Drawing for the job (mm, zero at the part's lowest x, y, z). A direction names the side the tool comes from. Round coordinates to 2 decimals unless told otherwise and drop trailing zeros. Write each loop counter-clockwise with the first axis right and the second up, starting at its lowest first coordinate (ties: lowest second). Pieces come first, ordered by that corner, then holes. Notation, with made-up numbers: (-33.5, -21) -> (23.5, -21) arc R11 cw to (23.5, -8) -> close; hole circle Ø5 at (-35, 40). An arc over 180 degrees is marked (long way). One line per question, with ' | ' between items.
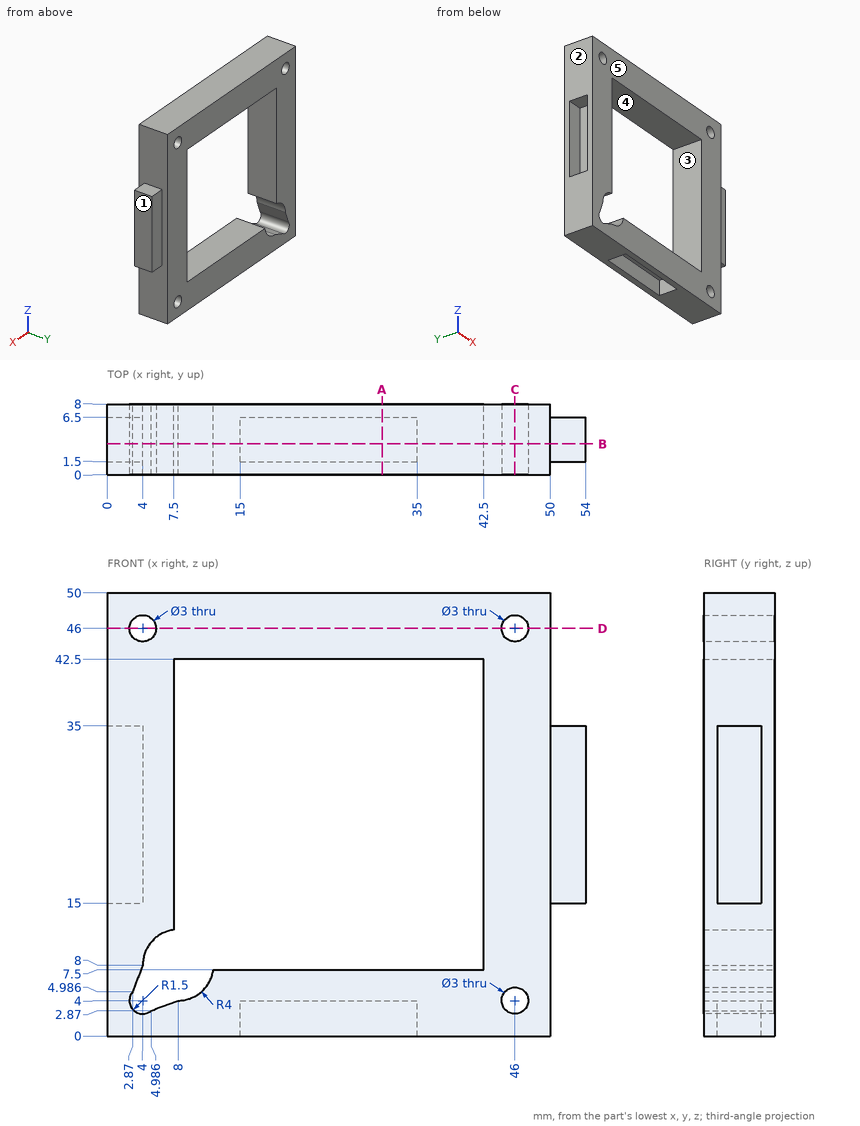
(1) Drop flat-ended pins along their axis: pin 1 (1.5 mm diameter, centred on y = 2, z = 13.5, fed in from +X); pin 2 (1.2 mm diameter, centred on x = 51, z = 29.5, fed in from +Y). Give the stop position or say it passes through.
Calculated:
pin 1: x = 50 | pin 2: y = 6.5
(2) Slice it at B-B (y = 3.5). Write the cut outline in (x, z), then the cut area to 3 significant figures.
Calculated:
outline: (0, 0) -> (15, 0) -> (15, 4) -> (35, 4) -> (35, 0) -> (50, 0) -> (50, 15) -> (54, 15) -> (54, 35) -> (50, 35) -> (50, 50) -> (0, 50) -> (0, 35) -> (4, 35) -> (4, 15) -> (0, 15) -> close; hole circle Ø3 at (4, 46); hole (2.87, 4.99) arc R1.5 ccw to (4.99, 2.87) -> (8, 4) arc R4 ccw to (11.97, 7.5) -> (42.5, 7.5) -> (42.5, 42.5) -> (7.5, 42.5) -> (7.5, 11.97) arc R4 ccw to (4, 8) -> close; hole circle Ø3 at (46, 4); hole circle Ø3 at (46, 46) | area: 1,130 mm2
(3) Wall check: line 1 (X direction, y = 5.5, z = 46); line 2 (X direction, y = 3.25, z = 39.5). Give the ranges that are in metal, low to high. Write a range as from..to.
Calculated:
line 1: 0..2.5, 5.5..44.5, 47.5..50 | line 2: 0..7.5, 42.5..50
(4) Mould opens along X. For the marked faces 1, 2 and 3 say: pulls with the +X half, pulls with the -X half, needs draft (parallel to the pull), parting line crosses it, or undercut.
Calculated:
face 1: pulls with the +X half | face 2: pulls with the -X half | face 3: undercut
(5) 3-axis set-ups, long thin cutter, end or side, ignore diameter. For the marked faces 4 and 5: which of +Z, -Z, +X, -X, +Y, -Y reach the whole face in a straight line?
Calculated:
face 4: +Y, -Y | face 5: +Z, -Z, +X, -X, -Y
(6) Slice it at A-A (x = 31). Write the cut outline in (y, z).
Calculated:
outline: (0, 0) -> (1.5, 0) -> (1.5, 4) -> (6.5, 4) -> (6.5, 0) -> (8, 0) -> (8, 7.5) -> (0, 7.5) -> close; (0, 42.5) -> (8, 42.5) -> (8, 50) -> (0, 50) -> close
(7) Slice it at C-C (x = 46). Write the cut outline in (y, z).
Calculated:
outline: (0, 0) -> (8, 0) -> (8, 2.5) -> (0, 2.5) -> close; (0, 5.5) -> (8, 5.5) -> (8, 44.5) -> (0, 44.5) -> close; (0, 47.5) -> (8, 47.5) -> (8, 50) -> (0, 50) -> close
(8) Slice it at D-D (z = 46). Write the cut outline in (x, y), then the cut area to 3 significant figures.
Calculated:
outline: (0, 0) -> (2.5, 0) -> (2.5, 8) -> (0, 8) -> close; (5.5, 0) -> (44.5, 0) -> (44.5, 8) -> (5.5, 8) -> close; (47.5, 0) -> (50, 0) -> (50, 8) -> (47.5, 8) -> close | area: 352 mm2
